Autodesk Inventor part; units mm, degrees
ref_plane "YZ Plane" through (0, 0, 0) normal (1, 0, 0) x (0, 1, 0)
ref_plane "XZ Plane" through (0, 0, 0) normal (0, 1, 0) x (-1, 0, 0)
ref_plane "XY Plane" through (0, 0, 0) normal (0, 0, 1) x (1, 0, 0)
sketch "Эскиз1" plane through (0, 0, 0) normal (1, 0, 0) x (0, 1, 0)
  line L0 (84, 90) -> (0, 90)
  line L1 (0, 90) -> (0, -90)
  line L2 (0, -90) -> (84, -90)
  line L3 (84, -90) -> (84, 90)
  line L4 (76, 90) -> (8, 90)
  line L5 (8, 90) -> (8, 96)
  line L6 (8, 96) -> (76, 96)
  line L7 (76, 96) -> (76, 90)
  line L8 (76, -90) -> (8, -90)
  line L9 (8, -90) -> (8, -96)
  line L10 (8, -96) -> (76, -96)
  line L11 (76, -96) -> (76, -90)
  line L12 (16, -96) -> (16, -90)
  line L13 (32, -96) -> (32, -90)
  line L14 (68, -96) -> (68, -90)
  line L15 (52, -96) -> (52, -90)
  line L16 (16, 90) -> (16, 96)
  line L17 (32, 90) -> (32, 96)
  line L18 (68, 90) -> (68, 96)
  line L19 (52, 90) -> (52, 96)
  circle A0 centre (20, -59.5) radius 1.5
  circle A1 centre (20, -73.5) radius 1.5
  circle A2 centre (7, -59.5) radius 1.5
  circle A3 centre (7, -73.5) radius 1.5
  line L20 (20, -59.5) -> (0, -59.5) construction
  line L21 (7, -59.5) -> (7, -73.5) construction
  line L22 (20, -73.5) -> (0, -73.5) construction
  point P0 (0, 0)
  point P1 (76, 93)
  point P2 (8, 93)
  point P3 (8, -90)
  point P4 (68, -93)
  point P5 (76, -93)
  point P6 (52, -93)
  point P7 (16, -93)
  point P8 (8, -93)
  point P9 (32, -93)
  point P10 (68, 93)
  point P11 (52, 93)
  point P12 (16, 93)
  point P13 (32, 93)
  dimension "d0" = 180
  dimension "d1" = 84
  dimension "d2" = 90
  dimension "d3" = 0
  dimension "d4" = 6
  dimension "d5" = 8
  dimension "d6" = 8
  dimension "d7" = 6
  dimension "d40" = 8
  dimension "d41" = 16
  dimension "d42" = 8
  dimension "d43" = 16
  dimension "d44" = 8
  dimension "d45" = 16
  dimension "d46" = 16
  dimension "d47" = 8
  dimension "d76" = 14
  dimension "d77" = 3
  dimension "d78" = 3
  dimension "d79" = 20
  dimension "d80" = 20
  dimension "d81" = 3
  dimension "d82" = 3
  dimension "d83" = 13
  dimension "d84" = 13
  dimension "d85" = 16.5
extrude "Выдавливание1" add sketch "Эскиз1" along normal blind 6 contours L3 L2 L1 L0 | L0 L18 L6 L7 | L11 L10 L14 L2 | L0 L17 L6 L19 | L15 L10 L13 L2 | L0 L5 L6 L16 | L12 L10 L9 L2 | A0 | A1 | A2 | A3
sketch "Эскиз4" plane through (0, 84, 90) normal (0, 1, 0) x (1, 0, 0)
  circle A0 centre (3, 5) radius 1.5
  circle A1 centre (3, 175) radius 1.5
  line L0 (0, 0) -> (6, 0)
  line L1 (6, 180) -> (6, 0)
  line L2 (0, 180) -> (6, 180)
  line L3 (6, 180) -> (6, 0)
  line L4 (0, 0) -> (6, 0)
  line L5 (0, 180) -> (6, 180)
  point P0 (0, 90)
  point P1 (3, 0)
  dimension "d30" = 3
  dimension "d31" = 3
  dimension "d32" = 5
  dimension "d33" = 3
  dimension "d34" = 5
  dimension "d35" = 3
  dimension "d36" = 6
  dimension "d37" = 6
extrude "Выдавливание4" cut sketch "Эскиз4" against normal blind 4
sketch "Эскиз6" plane through (6, 0, 0) normal (1, 0, 0) x (0, 0, -1)
  line L0 (-90, 8) -> (-90, 0)
  line L1 (-90, 0) -> (-70, 0)
  line L2 (-70, 0) -> (-70, -6)
  line L3 (-70, -6) -> (-90, -6)
  line L4 (-90, -6) -> (-90, 0)
  line L5 (-90, 0) -> (90, 0)
  line L6 (-50, 0) -> (-30, 0)
  line L7 (-30, 0) -> (-30, -6)
  line L8 (-30, -6) -> (-50, -6)
  line L9 (-50, -6) -> (-50, 0)
  line L10 (30, 0) -> (50, 0)
  line L11 (50, 0) -> (50, -6)
  line L12 (50, -6) -> (30, -6)
  line L13 (30, -6) -> (30, 0)
  line L14 (90, 0) -> (70, 0)
  line L15 (70, 0) -> (70, -6)
  line L16 (70, -6) -> (90, -6)
  line L17 (90, -6) -> (90, 0)
  point P0 (0, 0)
  point P1 (-80, -6)
  point P2 (-50, -3)
  point P3 (-70, -3)
  point P4 (-30, -3)
  point P5 (90, -3)
  point P6 (70, -3)
  point P7 (50, -3)
  dimension "d48" = 6
  dimension "d49" = 6
  dimension "d50" = 6
  dimension "d51" = 20
  dimension "d52" = 20
  dimension "d53" = 20
  dimension "d54" = 20
  dimension "d55" = 20
  dimension "d56" = 20
extrude "Выдавливание5" add sketch "Эскиз6" against normal blind 6
sketch "Эскиз8" plane through (6, 0, 0) normal (1, 0, 0) x (0, 0, -1)
  line L0 (90, 60) -> (80, 60)
  line L1 (80, 60) -> (80, 57)
  line L2 (80, 57) -> (90, 57)
  line L3 (90, 57) -> (90, 60)
  line L4 (85.6, 55.5) -> (88, 55.5)
  line L5 (88, 55.5) -> (88, 61.5)
  line L6 (88, 61.5) -> (85.6, 61.5)
  line L7 (85.6, 61.5) -> (85.6, 55.5)
  line L8 (90, 25.5) -> (80, 25.5)
  line L9 (80, 25.5) -> (80, 22.5)
  line L10 (80, 22.5) -> (90, 22.5)
  line L11 (90, 22.5) -> (90, 25.5)
  line L12 (85.6, 27) -> (88, 27)
  line L13 (88, 27) -> (88, 21)
  line L14 (88, 21) -> (85.6, 21)
  line L15 (85.6, 21) -> (85.6, 27)
  line L16 (-85.6, 27) -> (-88, 27)
  line L17 (-90, 22.5) -> (-90, 25.5)
  line L18 (-85.6, 21) -> (-85.6, 27)
  line L19 (-88, 21) -> (-85.6, 21)
  line L20 (-88, 27) -> (-88, 21)
  line L21 (-80, 61.5) -> (-80, 58.5)
  line L22 (-90, 61.5) -> (-80, 61.5)
  line L23 (-80, 25.5) -> (-80, 22.5)
  line L24 (-90, 25.5) -> (-80, 25.5)
  line L25 (-80, 22.5) -> (-90, 22.5)
  line L26 (-80, 58.5) -> (-90, 58.5)
  line L27 (-85.6, 57) -> (-88, 57)
  line L28 (-90, 58.5) -> (-90, 61.5)
  line L29 (-88, 57) -> (-88, 63)
  line L30 (-85.6, 63) -> (-85.6, 57)
  line L31 (-88, 63) -> (-85.6, 63)
  line L32 (90, 32) -> (96, 32)
  line L33 (90, 16) -> (90, 32)
  line L34 (90, 68) -> (96, 68)
  line L35 (-96, 68) -> (-90, 68)
  line L36 (-90, 68) -> (-90, 52)
  line L37 (-90, 32) -> (-90, 16)
  line L38 (-96, 32) -> (-90, 32)
  point P0 (0, 0)
  point P1 (97.0761, 73.2611)
  point P2 (97.0761, 37.2611)
  point P3 (-93, 32)
  point P4 (85.6, 22.5)
  point P5 (88, 22.5)
  point P6 (88, 25.5)
  point P7 (85.6, 25.5)
  point P8 (85.6, 57)
  point P9 (88, 57)
  point P10 (88, 60)
  point P11 (85.6, 60)
  point P12 (-88, 25.5)
  point P13 (-88, 22.5)
  point P14 (-85.6, 22.5)
  point P15 (-85.6, 25.5)
  point P16 (-85.6, 61.5)
  point P17 (-88, 61.5)
  point P18 (-88, 58.5)
  point P19 (-85.6, 58.5)
  dimension "d86" = 6
  dimension "d87" = 2.4
  dimension "d88" = 10
  dimension "d89" = 3
  dimension "d90" = 1.5
  dimension "d91" = 5.6
  dimension "d92" = 10
  dimension "d93" = 3
  dimension "d94" = 1.5
  dimension "d95" = 6
  dimension "d96" = 5.6
  dimension "d97" = 2.4
  dimension "d100" = 6.5
  dimension "d101" = 10
  dimension "d102" = 8
  dimension "d103" = 6.5
  dimension "d104" = 3
  dimension "d105" = 10
  dimension "d106" = 2.4
  dimension "d107" = 1.5
  dimension "d108" = 6
  dimension "d109" = 2
  dimension "d110" = 6
  dimension "d111" = 2.4
  dimension "d112" = 10
  dimension "d113" = 3
  dimension "d114" = 6.5
  dimension "d115" = 1.5
extrude "Выдавливание7" cut sketch "Эскиз8" against normal blind 10
properties part number "передняя стенка"
Verification items for the finished model (mm, model axes). A direction names the side the tool comes from. Coordinates: 2 decimals unless noted, no trailing zeros. Loops run counter-clockwise (first coordinate to the right, second up) from the corner with the lowest first, then second, coordinate; pieces in that order, holes last. Notation, with made-up numbers: (52.5, 77) - (92.5, 77) arc R24 ccw to (92.5, 91) - close; hole circle Ø5 at (50.5, 5). An arc over 180 degrees is marked (long way). Put each result on its own line as item: value.
Item 1: Gauge pin test, flat ends, axial feed: pin 1 Ø1.6 at (x, y) = (3.5, 22) entering from +Z; pin 2 Ø3 at (x, y) = (3.5, 63) entering from -Z; pin 3 Ø3 at (x, z) = (2.5, -94.5) entering from +Y. Record the tip position at first contact, or that the pin passes through.
Conclusion:
pin 1: stops at z = 90
pin 2: stops at z = -90
pin 3: stops at y = 76
Item 2: Draft check along Y on faces 5 (the face through (3, 68, 93)), 6 (the face through (3, 0, 0)), 7 (the face through (3, -3, -70)). Enter one of: pulls with the +Y half, pulls with the -Y half, needs draft (parallel to the pull), parting line crosses it, or undercut.
Conclusion:
face 5: undercut
face 6: pulls with the -Y half
face 7: needs draft
Item 3: Section check A-A (z = 18). Enter the section's corners in (x, y).
Conclusion:
outline: (0, 0) - (6, 0) - (6, 84) - (0, 84) - close
Item 4: Set-up check for faces 1 (the face through (3, 80, -90)), 2 (the face through (3, -3, -50)), 3 (the face through (3, 1, -90)), 4 (the face through (3, 54, -90)): record each of +Z, -Z, +X, -X, +Y, -Y from which the full face is reachable in a straight line by a thin tool's end or side.
Conclusion:
face 1: -Z, +X, -X, +Y
face 2: +X, -X, -Y
face 3: -Z, +X, -X, -Y
face 4: -Z, +X, -X
Item 5: Scan lines: line 1 along Z through (x, y) = (3, 81.85); line 2 along Y through (x, z) = (4.2, -83); line 3 along Y through (x, z) = (1.1, -86). Record each from-to range of solid material in increasing order.
Conclusion:
line 1: z = -90 to -86.5, -83.5 to 83.5, 86.5 to 90
line 2: y = -6 to 22.5, 25.5 to 57, 60 to 84
line 3: y = -6 to 21, 27 to 55.5, 61.5 to 84
